Autodesk Fusion 360 part; units mm, degrees
sketch "Sketch1" plane through (0, 0, 0) normal (0, 1, 0) x (1, 0, 0)
  line L0 (-12.5, -96.75) -> (-12.5, 96.75)
  line L1 (12.5, 96.75) -> (12.5, -96.75)
  circle A0 centre (0, -96.75) radius 9.25
  arc A1 (-12.5, -96.75) -> (12.5, -96.75) centre (0, -96.75) ccw
  circle A2 centre (0, 96.75) radius 9.25
  arc A3 (12.5, 96.75) -> (-12.5, 96.75) centre (0, 96.75) ccw
extrude "Extrude1" add sketch "Sketch1" along normal blind 6
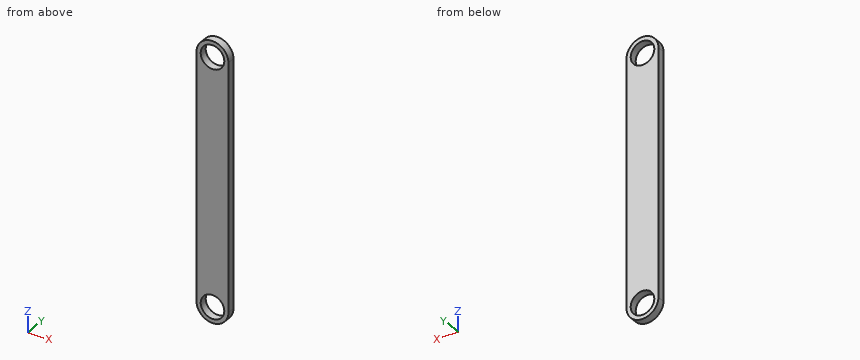
Check sheet for the modelled part. Datum: model origin and axes. Units: mm. Give positions to 0.01 mm unless a question says otherwise; leave off trailing zeros. Write each loop counter-clockwise with the first axis right and the second up, starting at its lowest first coordinate (ties: lowest second). Pieces come first, ordered by that corner, then holes. Notation, with made-up numbers: (73.5, 10) -> (129.5, 10) arc R32 cw to (129.5, 44) -> close; hole circle Ø6 at (71.25, 54). An arc over 180 degrees is marked (long way). Write item = value, one per line.
Item 1: Sectioned sample at A-A on x = 0. Record the boundary of the cut face in (y, z).
Output:
outline = (0, -109.25) -> (6, -109.25) -> (6, -106) -> (0, -106) -> close; (0, -87.5) -> (6, -87.5) -> (6, 87.5) -> (0, 87.5) -> close; (0, 106) -> (6, 106) -> (6, 109.25) -> (0, 109.25) -> close
Item 2: Scan lines: probe 1 along Z at (x, y) = (0, 4.7); probe 2 along X at (y, z) = (2.9, -96.75); probe 3 along Z at (x, y) = (-7.25, 2.1). Record each from-to range of solid material in increasing order. Write a range as from..to.
Output:
probe_1 = -109.25..-106, -87.5..87.5, 106..109.25
probe_2 = -12.5..-9.25, 9.25..12.5
probe_3 = -106.93..-102.49, -91.01..91.01, 102.49..106.93
Item 3: Sectioned sample at B-B on y = 4.9. Record the boundary of the cut face in (x, z).
Output:
outline = (-12.5, -96.75) arc R12.5 ccw to (12.5, -96.75) -> (12.5, 96.75) arc R12.5 ccw to (-12.5, 96.75) -> close; hole circle Ø18.5 at (0, -96.75); hole circle Ø18.5 at (0, 96.75)
